```python
from build123d import *

# Parameters (mm, degrees)
F0_W     = 88.9
F0_H     = 190.5
F1_DEPTH = 2260.6


with BuildPart() as f1:
    # F0 (on Front) → F1 (new body)
    with BuildSketch(Plane.XZ):
        with BuildLine():
            Line((42.300776, 102.158077), (-46.599224, 102.158077))
            ThreePointArc((-46.599224, 102.158077), (-51.089352, 100.298206), (-52.949224, 95.808077))
            Line((-52.949224, 95.808077), (-52.949224, -94.691923))
            ThreePointArc((-52.949224, -94.691923), (-51.089352, -99.182051), (-46.599224, -101.041923))
            Line((-46.599224, -101.041923), (42.300776, -101.041923))
            ThreePointArc((42.300776, -101.041923), (46.790904, -99.182051), (48.650776, -94.691923))
            Line((48.650776, -94.691923), (48.650776, 95.808077))
            ThreePointArc((48.650776, 95.808077), (46.790904, 100.298206), (42.300776, 102.158077))
        make_face()
        with Locations((-2.149224, 0.558077)):
            Rectangle(F0_W, F0_H, mode=Mode.SUBTRACT)
    extrude(amount=F1_DEPTH)


solid = f1.part
```
Check sheet for the modelled part. Datum: model origin and axes. Units: mm. A direction names the side the tool comes from. Round coordinates to 2 decimals unless told otherwise and drop trailing zeros. Loops run counter-clockwise (first coordinate to the right, second up) from the corner with the lowest first, then second, coordinate; pieces in that order, holes last. Notation, with made-up numbers: (66.25, 87.5) - (104.25, 87.5) arc R20 ccw to (104.25, 125.5) - close; hole circle Ø3 at (85, 37.5). An arc over 180 degrees is marked (long way). Write item = value, one per line. Start each with the question number.
Q1. Access from +Z, -Z, +X, -X, +Y, -Y to the whole of each face (thin tool, end or side, straight path). Record for faces 4 (the face through (42.301, -1114, -1)), 5 (the face through (-3, -1114, -101.042)).
Q2. Section check B-B (z = -25). Record the boundary of the cut face in (x, y), plus the area to 3 significant figures.
Q3. Section check C-C (y = -590). Record the boundary of the cut face in (x, z).
Q4. Section check A-A (x = 3). Record the boundary of the cut face in (y, z), plus the area to 3 significant figures.
Q5. Thickness scan on L1, parallel to Z at x = 24, y = -2105; L2, parallel to X at y = -1715.5, z = 73.5; L3, parallel to Z at x = 44.5, y = -2113. Record the ranges inside material, lowest first.
Q6. Release check for a two-part mould opening along Z. For faces 1 (the face through (-2, -1114, 102.158)), 2 (the face through (-52.949, -1114, 2)), 3 (the face through (-3, -1114, 95.808)) record: pulls with the +Z half, pulls with the -Z half, needs draft (parallel to the pull), parting line crosses it, or undercut.
Derived:
q1.face_4 = +Y, -Y
q1.face_5 = -Z, +X, -X, +Y, -Y
q2.outline = (-52.95, -2260.6) - (-46.6, -2260.6) - (-46.6, 0) - (-52.95, 0) - close; (42.3, -2260.6) - (48.65, -2260.6) - (48.65, 0) - (42.3, 0) - close
q2.area = 28,700 mm^2
q3.outline = (-52.95, -94.69) arc R6.35 ccw to (-46.6, -101.04) - (42.3, -101.04) arc R6.35 ccw to (48.65, -94.69) - (48.65, 95.81) arc R6.35 ccw to (42.3, 102.16) - (-46.6, 102.16) arc R6.35 ccw to (-52.95, 95.81) - close; hole (-46.6, -94.69) - (42.3, -94.69) - (42.3, 95.81) - (-46.6, 95.81) - close
q4.outline = (-2260.6, -101.04) - (0, -101.04) - (0, -94.69) - (-2260.6, -94.69) - close; (-2260.6, 95.81) - (0, 95.81) - (0, 102.16) - (-2260.6, 102.16) - close
q4.area = 28,700 mm^2
q5.L1 = -101.04 to -94.69, 95.81 to 102.16
q5.L2 = -52.95 to -46.6, 42.3 to 48.65
q5.L3 = -100.65 to 101.77
q6.face_1 = pulls with the +Z half
q6.face_2 = needs draft
q6.face_3 = undercut
